Autodesk Inventor part; units mm, degrees
ref_plane "YZ Plane" through (0, 0, 0) normal (1, 0, 0) x (0, 1, 0)
ref_plane "XZ Plane" through (0, 0, 0) normal (0, 1, 0) x (-1, 0, 0)
ref_plane "XY Plane" through (0, 0, 0) normal (0, 0, 1) x (1, 0, 0)
sketch "Sketch1" plane through (0, 0, 0) normal (0, 0, 1) x (1, 0, 0)
  line L0 (22.5, 15) -> (-22.5, 15) construction
  line L1 (-22.5, 15) -> (-22.5, -15)
  line L2 (-22.5, -15) -> (22.5, -15)
  line L3 (22.5, -15) -> (22.5, 15)
  line L4 (22.5, 15) -> (-22.5, -15) construction
  line L5 (-22.5, 15) -> (22.5, -15) construction
  line L6 (-27.5, -20) -> (-27.5, 15)
  line L7 (-27.5, 20) -> (27.5, 20) construction
  line L8 (27.5, 20) -> (27.5, 15) construction
  line L9 (27.5, -20) -> (-27.5, -20)
  line L10 (-22.5, 15) -> (-27.5, 15)
  line L11 (22.5, 15) -> (27.5, 15)
  line L12 (-27.5, 15) -> (-27.5, 20) construction
  line L13 (27.5, 15) -> (27.5, -20)
  point P0 (0, 0)
  dimension "d0" = 45
  dimension "d1" = 30
  dimension "d2" = 5
  dimension "d3" = 5
  dimension "d4" = 5
  dimension "d5" = 40
extrude "Extrusion1" add sketch "Sketch1" along normal blind 20
properties part number "track z2043"
Read the model definition and answer for the solid it produces. Units are mm, in the model's axes. A direction names the side the tool comes from. Round coordinates to 2 decimals unless told otherwise and drop trailing zeros. Write each loop counter-clockwise with the first axis right and the second up, starting at its lowest first coordinate (ties: lowest second). Pieces come first, ordered by that corner, then holes. Notation, with made-up numbers: M 66.25,6 L 108.25,6 A12 ccw 108.25,25 Z; hole C 4,27 d2. An arc over 180 degrees is marked long. Use a Markdown table: item, result.
1) A flat-ended cylindrical pin translates along its axis: pin 1 (6 mm diameter, centred on x = -5, z = 2.5, fed in from +Y). Find the tip coordinate at first contact, or state that the pin passes through.
Answers follow:
| item | result |
|---|---|
| pin 1 | stops at y = -15 |
2) Straight lines are drawn through the part: line 1 along X through (y, z) = (3, 5.5); line 2 along Y through (x, z) = (1.5, 8.5). For each, find the intervals that lie inside material, in ascending order. Write a range as [from, to].
Answers follow:
| item | result |
|---|---|
| line 1 | x = [-27.5, -22.5], [22.5, 27.5] |
| line 2 | y = [-20, -15] |
3) The part is cut by section A-A (y = -14). Write down the section's boundary in (x, z), plus the area to 3 significant figures.
Answers follow:
| item | result |
|---|---|
| outline | M -27.5,0 L -22.5,0 L -22.5,20 L -27.5,20 Z; M 22.5,0 L 27.5,0 L 27.5,20 L 22.5,20 Z |
| area | 200 mm2 |
4) For a pull along X with two mould halves and no side action, classify faces 1 (the flat face through (27.5, -2, 10)), 2 (the flat face through (0, -15, 10)), 3 (the flat face through (25, 15, 10)) as pulls with the +X half, pulls with the -X half, needs draft (parallel to the pull), parting line crosses it, or undercut.
Answers follow:
| item | result |
|---|---|
| face 1 | pulls with the +X half |
| face 2 | undercut |
| face 3 | needs draft |
5) A tool of negligible diameter and unlimited length cuts with its end or side. For faces 4 (the flat face through (-0.1, -15.4, 0)), 5 (the flat face through (-22.5, 0, 10)), from which of +Z, -Z, +X, -X, +Y, -Y can it reach the whole face along a straight path? Write none if from no direction.
Answers follow:
| item | result |
|---|---|
| face 4 | -Z, +X, -X, +Y, -Y |
| face 5 | +Z, -Z, +Y |
6) The part is cut by section C-C (x = 19). Write down the section's boundary in (y, z).
Answers follow:
| item | result |
|---|---|
| outline | M -20,0 L -15,0 L -15,20 L -20,20 Z |
7) The part is cut by section B-B (z = 6). Write down the section's boundary in (x, y), plus the area to 3 significant figures.
Answers follow:
| item | result |
|---|---|
| outline | M -27.5,-20 L 27.5,-20 L 27.5,15 L 22.5,15 L 22.5,-15 L -22.5,-15 L -22.5,15 L -27.5,15 Z |
| area | 575 mm2 |
